Build history of the part. All positions in model axes, mm. A direction names the side the tool comes from. Round coordinates to 2 decimals unless told otherwise and drop trailing zeros. Write each loop counter-clockwise with the first axis right and the second up, starting at its lowest first coordinate (ties: lowest second). Pieces come first, ordered by that corner, then holes. Notation, with made-up numbers: (9, 70) - (66, 70) arc R19 cw to (66, 89) - close; hole circle Ø11 at (-39.75, -2). An arc over 180 degrees is marked (long way). Answer as a JSON object with one key per item and string values. Group by question number.
Item 1: Flat gauge pins, fed straight in: pin 1 (1.9 mm diameter, centred on x = -103.5, y = -2, fed in from -Z); pin 2 (1.5 mm diameter, centred on x = 17, y = -3.5, fed in from +Z); pin 3 (3 mm diameter, centred on y = -2, z = -13, fed in from -X). Where does each tip first touch, or does it go through?
Item 2: Slice it at D-D, the plane y = -4.75. Give the number of separate pieces and of enclosed holes in the cut face, then the cut area to 3 significant figures.
Item 3: Probe line 1 (X direction, y = -4.5, z = 6); line 2 (X direction, y = -4, z = 37.5); line 3 (Z direction, x = -95, y = -3.25). List the from-to ranges inside material, lowest first. Write a range as from..to.
Item 4: Two-plate mould, pull along Z, no slides. Class faces 1 (the cylindrical face through (15.815, -3.131, -16.709)), 2 (the cylindrical face through (0.2, -3.1, -62.5)), 3 (the flat face through (10, -3, -47)), 4 (the cylindrical face through (-133.57, -3.13, 5.38)): +Z half, -Z half, draft (parallel to the pull), parting line (faces both ways), or undercut.
Item 5: Slice it at B-B, the plane x = -104.5. List the corners of the cut face in (y, z), then the cut area to 3 significant figures.
Item 6: Slice it at C-C, the plane z = 37.5. List the corners of the cut face in (x, y).
Item 7: Slice it at A-A, the plane z = 0. List the corners of the cut face in (x, y).
Item 8: Which spindle directions (+Z, -Z, +X, -X, +Y, -Y) get a long thin tool onto all of the face, cutting with end or side? Do faces 5 (the cylindrical face through (-140.581, -3.131, -39.048)), 6 (the flat face through (-10, -3, -48)). Say none if no direction does.
from build123d import *

# Parameters (mm, degrees)
SKETCH1_R           = 2.1
SKETCH1_R_2         = 10
SKETCH1_R_3         = 2.5
BOSS_EXTRUDE1_DEPTH = 6.35


with BuildPart() as part:
    # Sketch1 → Boss-Extrude1 (new body)
    with BuildSketch(Plane(origin=(0, 0, 0), x_dir=(1, 0, 0), z_dir=(0, 1, 0))):
        with BuildLine():
            Line((-10, 42.5), (-142, 42.5))
            ThreePointArc((-142, 42.5), (-184.5, 0), (-142, -42.5))
            Line((-142, -42.5), (0, -42.5))
            ThreePointArc((0, -42.5), (42.200640469, -5.0354686), (10, 41.306779105))
            Line((10, 41.306779105), (10, 52.5))
            ThreePointArc((10, 52.5), (0, 62.5), (-10, 52.5))
            Line((-10, 52.5), (-10, 42.5))
        make_face()
        with Locations(Location((-104.5, 0, 0), (0, 0, 270))):
            Circle(SKETCH1_R, mode=Mode.SUBTRACT)
        with Locations(Location((-142, 37.5, 0), (0, 0, 270))):
            Circle(SKETCH1_R, mode=Mode.SUBTRACT)
        with Locations(Location((-142, -37.5, 0), (0, 0, 270))):
            Circle(SKETCH1_R, mode=Mode.SUBTRACT)
        with Locations(Location((-179.5, 0, 0), (0, 0, 270))):
            Circle(SKETCH1_R, mode=Mode.SUBTRACT)
        with Locations(Location((-142, 0, 0), (0, 0, 270))):
            Circle(SKETCH1_R_2, mode=Mode.SUBTRACT)
        with Locations(Location((0, 37.5, 0), (0, 0, 270))):
            Circle(SKETCH1_R, mode=Mode.SUBTRACT)
        with Locations(Location((17.67766953, 17.67766953, 0), (0, 0, 270))):
            Circle(SKETCH1_R, mode=Mode.SUBTRACT)
        with Locations(Location((-17.67766953, -17.67766953, 0), (0, 0, 270))):
            Circle(SKETCH1_R, mode=Mode.SUBTRACT)
        with Locations(Location((0, -37.5, 0), (0, 0, 270))):
            Circle(SKETCH1_R, mode=Mode.SUBTRACT)
        with Locations(Location((17.67766953, -17.67766953, 0), (0, 0, 270))):
            Circle(SKETCH1_R, mode=Mode.SUBTRACT)
        with Locations(Location((-37.5, 0, 0), (0, 0, 270))):
            Circle(SKETCH1_R, mode=Mode.SUBTRACT)
        with Locations(Location((0, 0, 0), (0, 0, 270))):
            Circle(SKETCH1_R_2, mode=Mode.SUBTRACT)
        with Locations(Location((37.5, 0, 0), (0, 0, 270))):
            Circle(SKETCH1_R, mode=Mode.SUBTRACT)
        with Locations(Location((-17.67766953, 17.67766953, 0), (0, 0, 270))):
            Circle(SKETCH1_R, mode=Mode.SUBTRACT)
        with Locations(Location((0, 52.5, 0), (0, 0, 270))):
            Circle(SKETCH1_R_3, mode=Mode.SUBTRACT)
    extrude(amount=-BOSS_EXTRUDE1_DEPTH)


solid = part.part
Geometry says:
{
 "1": {"pin 1": "stops at z = -42.5", "pin 2": "stops at z = 39.27", "pin 3": "stops at x = -182.91"},
 "2": {"separate pieces": "1", "enclosed holes": "15", "area": "17,300 mm^2"},
 "3": {"line 1": "x = -184.07..-150, -134..-8, 8..42.07", "line 2": "x = -162..-144.1, -139.9..-2.1, 2.1..20", "line 3": "z = -42.5..42.5"},
 "4": {"face 1": "undercut", "face 2": "-Z half", "face 3": "draft", "face 4": "undercut"},
 "5": {"outline": "(-6.35, -42.5) - (0, -42.5) - (0, -2.1) - (-6.35, -2.1) - close; (-6.35, 2.1) - (0, 2.1) - (0, 42.5) - (-6.35, 42.5) - close", "area": "513 mm^2"},
 "6": {"outline": "(-162, -6.35) - (-144.1, -6.35) - (-144.1, 0) - (-162, 0) - close; (-139.9, -6.35) - (-2.1, -6.35) - (-2.1, 0) - (-139.9, 0) - close; (2.1, -6.35) - (20, -6.35) - (20, 0) - (2.1, 0) - close"},
 "7": {"outline": "(-184.5, -6.35) - (-181.6, -6.35) - (-181.6, 0) - (-184.5, 0) - close; (-177.4, -6.35) - (-152, -6.35) - (-152, 0) - (-177.4, 0) - close; (-132, -6.35) - (-106.6, -6.35) - (-106.6, 0) - (-132, 0) - close; (-102.4, -6.35) - (-39.6, -6.35) - (-39.6, 0) - (-102.4, 0) - close; (-35.4, -6.35) - (-10, -6.35) - (-10, 0) - (-35.4, 0) - close; (10, -6.35) - (35.4, -6.35) - (35.4, 0) - (10, 0) - close; (39.6, -6.35) - (42.5, -6.35) - (42.5, 0) - (39.6, 0) - close"},
 "8": {"face 5": "+Y, -Y", "face 6": "-Z, -X, +Y, -Y"}
}
